Here's how the part is built. I have some questions about the finished solid (model axes, mm). A direction names the side the tool comes from. Give positions to 0.01 mm unless a question says otherwise; leave off trailing zeros. Write each loop counter-clockwise with the first axis right and the second up, starting at its lowest first coordinate (ties: lowest second). Pieces come first, ordered by that corner, then holes. Notation, with made-up numbers: (63, 12) -> (109, 12) arc R16 ccw to (109, 32) -> close; hole circle Ø1 at (61.25, 88.5). An arc over 180 degrees is marked (long way). Use one line per item in the form item = value.
```python
from build123d import *

# Parameters (mm, degrees)
F0_R     = 34.925
F0_R_2   = 7.9375
F1_DEPTH = 1.905
F3_DEPTH = 12.7
F8_DEPTH = 0.508
F9_R     = 0.50799


# Not quite as in the source:
# - a fillet or chamfer is up to 0.001 mm smaller than in the source, because OpenCascade refuses the exact size


with BuildPart() as f1:
    # F0 (on Front) → F1 (new body)
    with BuildSketch(Plane.XZ):
        Circle(F0_R)
        with BuildLine():
            ThreePointArc((7.9375, -20.6375), (-5.6126600757, -26.2501600757), (0, -12.7))
            ThreePointArc((0, -12.7), (5.6126600757, -15.0248399243), (7.9375, -20.6375))
        make_face(mode=Mode.SUBTRACT)
        with Locations((-20.6375, 0)):
            Circle(F0_R_2, mode=Mode.SUBTRACT)
        Polygon((-1.016, 0), (-1.016, 0.508), (0, 0.508), (1.016, 0.508), (1.016, 0), (1.016, -0.508), (0, -0.508), (-1.016, -0.508), align=None, mode=Mode.SUBTRACT)
        with BuildLine():
            ThreePointArc((28.575, 0), (20.6375, -7.9375), (12.7, 0))
            ThreePointArc((12.7, 0), (20.6375, 7.9375), (28.575, 0))
        make_face(mode=Mode.SUBTRACT)
        with BuildLine():
            ThreePointArc((7.9375, 20.6375), (5.6126600757, 15.0248399243), (0, 12.7))
            ThreePointArc((0, 12.7), (-5.6126600757, 26.2501600757), (7.9375, 20.6375))
        make_face(mode=Mode.SUBTRACT)
    extrude(amount=F1_DEPTH)

    # F2 (on face) → F3 (join)
    with BuildSketch(Plane.XZ.offset(1.905)):
        with BuildLine():
            Line((-7.217116123, 23.9416097315), (-8.0497858212, 29.3670302556))
            ThreePointArc((-8.0497858212, 29.3670302556), (-11.0603471299, 16.316334461), (0, 8.763))
            Line((0, 8.763), (0, 12.7))
            ThreePointArc((0, 12.7), (-3.2253143504, 13.384827831), (-5.894084441, 15.3211408274))
            ThreePointArc((-5.894084441, 15.3211408274), (-7.8456367548, 19.4333861511), (-7.217116123, 23.9416097315))
        make_face()
        with BuildLine():
            Line((-23.5666824339, -7.3772485737), (-29.061654765, -8.3688330575))
            ThreePointArc((-29.061654765, -8.3688330575), (-16.1114020949, -10.9780776097), (-8.763, 0))
            Line((-8.763, 0), (-12.7, 0))
            ThreePointArc((-12.7, 0), (-13.3830221995, -3.2212510135), (-15.3145406216, -5.8881244642))
            ThreePointArc((-15.3145406216, -5.8881244642), (-19.2279203931, -7.8113373747), (-23.5666824339, -7.3772485737))
        make_face()
        with BuildLine():
            Line((23.9903295305, 7.1946118999), (29.4060203782, 8.0072967115))
            ThreePointArc((29.4060203782, 8.0072967115), (16.3432040729, 11.0708072308), (8.763, 0))
            Line((8.763, 0), (12.7, 0))
            ThreePointArc((12.7, 0), (13.384689213, 3.225002626), (15.3206341891, 5.8936274228))
            ThreePointArc((15.3206341891, 5.8936274228), (19.4595781944, 7.8496118675), (23.9903295305, 7.1946118999))
        make_face()
        with BuildLine():
            Line((7.374412056, -23.5738162429), (8.3621654342, -29.0682733631))
            ThreePointArc((8.3621654342, -29.0682733631), (10.9798672248, -16.1157452549), (0, -8.763))
            Line((0, -8.763), (0, -12.7))
            ThreePointArc((0, -12.7), (3.2225232211, -13.3835872393), (5.8899911345, -15.3166062137))
            ThreePointArc((5.8899911345, -15.3166062137), (7.4079589254, -17.786877119), (7.9375, -20.6375))
            ThreePointArc((7.9375, -20.6375), (7.7954570727, -22.1324097892), (7.374412056, -23.5738162429))
        make_face()
    extrude(amount=F3_DEPTH)

    # F4 (on face) + F7 (on face) + F6 (on face) + F5 (on face) → F8 (join)
    with BuildSketch(Plane.XZ.offset(14.605)):
        with BuildLine():
            Line((-12.7, 0), (-20.6375, 0))
            Line((-20.6375, 0), (-23.5666824339, 0))
            Line((-23.5666824339, 0), (-23.5666824339, -7.3772485737))
            ThreePointArc((-23.5666824339, -7.3772485737), (-16.1791639494, -6.567126153), (-12.7, 0))
        make_face()
        Polygon((-23.5666824339, -7.3772485737), (-23.5666824339, 0), (-29.061654765, 0), (-29.061654765, -8.3688330575), align=None)
    with BuildSketch(Plane.XZ.offset(14.605)):
        with BuildLine():
            Line((0, 23.9416097315), (-7.217116123, 23.9416097315))
            ThreePointArc((-7.217116123, 23.9416097315), (-6.6794564616, 16.3492873621), (0, 12.7))
            Line((0, 12.7), (0, 20.6375))
            Line((0, 20.6375), (0, 23.9416097315))
        make_face()
        Polygon((-8.0497858212, 29.3670302556), (-7.217116123, 23.9416097315), (0, 23.9416097315), (0, 29.3670302556), align=None)
    with BuildSketch(Plane.XZ.offset(14.605)):
        with BuildLine():
            ThreePointArc((23.9903295305, 7.1946118999), (16.3718920801, 6.6939147981), (12.7, 0))
            Line((12.7, 0), (20.6375, 0))
            Line((20.6375, 0), (23.9903295305, 0))
            Line((23.9903295305, 0), (23.9903295305, 7.1946118999))
        make_face()
        Polygon((29.4060203782, 8.0072967115), (23.9903295305, 7.1946118999), (23.9903295305, 0), (29.4060203782, 0), align=None)
    with BuildSketch(Plane.XZ.offset(14.605)):
        with BuildLine():
            Line((0, -12.7), (0, -20.6375))
            Line((0, -20.6375), (0, -23.5738162429))
            Line((0, -23.5738162429), (7.374412056, -23.5738162429))
            ThreePointArc((7.374412056, -23.5738162429), (6.5692814077, -16.1823402906), (0, -12.7))
        make_face()
        Polygon((7.374412056, -23.5738162429), (0, -23.5738162429), (0, -29.0682733631), (8.3621654342, -29.0682733631), align=None)
    extrude(amount=-F8_DEPTH)

    # F9 (radius 0.508 in the source; OpenCascade refuses exactly that, so slightly less here)
    f9_edges = [f1.edges().sort_by_distance(p)[0] for p in [
        (1.016, -0.9525, 0.508),
        (1.016, -0.9525, -0.508),
        (-1.016, -0.9525, -0.508),
        (-1.016, -0.9525, 0.508),
    ]]
    fillet(f9_edges, radius=F9_R)


solid = f1.part
```
Q1. I want a section at D-D, the plane z = 19. Write out the boundary of the cut face in (x, y) (3 decimals), and give its area (3 significant figures).
Result set:
outline = (-29.305, -1.905) -> (-11.761, -1.905) -> (-11.761, -14.605) -> (0, -14.605) -> (0, -14.097) -> (-7.767, -14.097) -> (-7.767, 0) -> (-29.305, 0) -> close; (7.767, -1.905) -> (29.305, -1.905) -> (29.305, 0) -> (7.767, 0) -> close
area = 137 mm2
Q2. I want a section at C-C, the plane z = -4.5. Write out the boundary of the cut face in (x, y) (3 decimals), and give its area (3 significant figures).
Result set:
outline = (-34.634, -1.905) -> (-27.176, -1.905) -> (-27.176, 0) -> (-34.634, 0) -> close; (-29.062, -14.605) -> (-9.649, -14.605) -> (-9.649, -1.905) -> (14.099, -1.905) -> (14.099, 0) -> (-14.099, 0) -> (-14.099, -14.097) -> (-29.062, -14.097) -> close; (27.176, -1.905) -> (34.634, -1.905) -> (34.634, 0) -> (27.176, 0) -> close
area = 146 mm2
Q3. If we mould it in two halves opening along Z, with no side actions, what happens to faces 4 (the face through (26.7, -7.9, 7.6)), 5 (the face through (12, -9, 0)), 6 (the face through (19, -14.605, 5))? For each: +Z half, -Z half, draft (parallel to the pull), parting line (faces both ways), or undercut.
Result set:
face_4 = -Z half
face_5 = undercut
face_6 = draft
Q4. I want a section at A-A, the plane y = -12.75. Write out the boundary of the cut face in (x, z) (1 decimal), and give its area (3 significant figures).
Result set:
outline = (-29.1, -8.4) arc R11.9 ccw to (-8.8, 0) -> (-12.7, 0) arc R7.9 cw to (-23.6, -7.4) -> close; (-8, 29.4) arc R11.9 ccw to (0, 8.8) -> (0, 12.7) arc R7.9 cw to (-7.2, 23.9) -> close; (0, -12.7) arc R7.9 cw to (7.4, -23.6) -> (8.4, -29.1) arc R11.9 ccw to (0, -8.8) -> close; (8.8, 0) -> (12.7, 0) arc R7.9 cw to (24, 7.2) -> (29.4, 8) arc R11.9 ccw to start
area = 348 mm2
Q5. Will these pins go through, and if not, where does the flat tip stop? pin 1 Ø1.1 at (x, y) = (0, -1) entering from -Z (3 decimals); pin 2 Ø1.5 at (x, y) = (5.5, -2.5) entering from -Z; pin 3 Ø1 at (x, z) = (23, -27) entering from +Y; pin 4 Ø6 at (y, z) = (-12, -2) entering from +X.
Result set:
pin_1 = -34.925
pin_2 = -34.56
pin_3 = through
pin_4 = 29.41
Q6. Which directions (+Z, -Z, +X, -X, +Y, -Y) give clear straight access to the entire face, cutting with the end or side of a thin tool? Please do faces 1 (the face through (7.86, -7.92, -26.28)), 2 (the face through (-7.63, -7.92, 26.62)), 3 (the face through (-11.13, -8.17, 16.5)).
Result set:
face_1 = -Z, -X
face_2 = +Z, +X
face_3 = -X, -Y
Q7. I want a section at B-B, the plane z = -18.5. Write out the boundary of the cut face in (x, y) (3 decimals), and give its area (3 significant figures).
Result set:
outline = (-29.623, -1.905) -> (-7.644, -1.905) -> (-7.644, 0) -> (-29.623, 0) -> close; (0, -14.605) -> (11.681, -14.605) -> (11.681, -1.905) -> (29.623, -1.905) -> (29.623, 0) -> (7.644, 0) -> (7.644, -14.097) -> (0, -14.097) -> close
area = 139 mm2
Q8. If I drill on line 1 along Z through (x, y) = (0, -0.45) (3 decimals); line 2 along Y through (x, z) = (2, -28.5) (3 decimals); line 3 along Z through (x, y) = (17, -1.25), over which ranges is the centre line in solid material (lowest first)? Write a range as from..to.
Result set:
line_1 = -34.925..-28.575, -12.7..-0.508, 0.508..12.7, 28.575..34.925
line_2 = -14.605..-14.097, -1.905..0
line_3 = -30.51..-7.05, 7.05..30.51
